from build123d import *

# Parameters (mm, degrees)
SKETCH1_W           = 72
SKETCH1_H           = 72
BOSS_EXTRUDE1_DEPTH = 15
SKETCH4_W           = 32
SKETCH4_H           = 64
CUT_EXTRUDE1_DEPTH  = 30
SKETCH8_R           = 10
SKETCH8_R_2         = 6
BOSS_EXTRUDE2_DEPTH = 10
BOSS_EXTRUDE3_DEPTH = 2


with BuildPart() as part:
    # Sketch1 → Boss-Extrude1 (new, symmetric)
    with BuildSketch(Plane.XY):
        with Locations((36, 36)):
            Rectangle(SKETCH1_W, SKETCH1_H)
    extrude(amount=BOSS_EXTRUDE1_DEPTH, both=True)

    # Sketch4 → Cut-Extrude1 (cut)
    with BuildSketch(Plane.XY.offset(15)):
        with Locations((56, 40)):
            Rectangle(SKETCH4_W, SKETCH4_H)
        with Locations((16, 40)):
            Rectangle(SKETCH4_W, SKETCH4_H)
    extrude(amount=-CUT_EXTRUDE1_DEPTH, mode=Mode.SUBTRACT)

    # Sketch8 → Boss-Extrude2 (add)
    with BuildSketch(Plane(origin=(0, 8, 0), x_dir=(1, 0, 0), z_dir=(0, 1, 0))):
        with Locations((18, 0)):
            Circle(SKETCH8_R)
        with Locations(Location((18, 0, 0), (0, 0, 180))):
            Circle(SKETCH8_R_2, mode=Mode.SUBTRACT)
    extrude(amount=BOSS_EXTRUDE2_DEPTH)

    # Sketch10 → Boss-Extrude3 (add, symmetric)
    with BuildSketch(Plane.XY):
        Polygon((40, 56), (54, 8), (72, 8), (72, 0), (0, 0), (0, 8), (32, 8), (32, 72), (40, 72), align=None)
    extrude(amount=BOSS_EXTRUDE3_DEPTH, both=True)


solid = part.part
CAD build for the part. Positions are in the model's coordinates, mm. A direction names the side the tool comes from. Give positions to 0.01 mm unless a question says otherwise; leave off trailing zeros. Loops run counter-clockwise (first coordinate to the right, second up) from the corner with the lowest first, then second, coordinate; pieces in that order, holes last. Notation, with made-up numbers: M -9.5,67.5 L 5.5,67.5 A18 cw 5.5,84.5 Z; hole C -1,-7.5 d8. An arc over 180 degrees is marked long. Write each question's results on one line, items separated by ' | '.
Q1. Band-saw the part on D-D on y = 61.5. Write the cut outline in (x, z).
Geometry check:
outline: M 32,-15 L 40,-15 L 40,15 L 32,15 Z
Q2. Band-saw the part on B-B on z = 0. Write the cut outline in (x, y).
Geometry check:
outline: M 0,0 L 72,0 L 72,8 L 54,8 L 40,56 L 40,72 L 32,72 L 32,8 L 28,8 L 28,18 L 24,18 L 24,8 L 12,8 L 12,18 L 8,18 L 8,8 L 0,8 Z
Q3. Band-saw the part on C-C on x = 18. Write the cut outline in (y, z).
Geometry check:
outline: M 0,-15 L 8,-15 L 8,-10 L 18,-10 L 18,-6 L 8,-6 L 8,6 L 18,6 L 18,10 L 8,10 L 8,15 L 0,15 Z
Q4. Flat gauge pins, fed straight in: P1, Ø9, axis at y = 53, z = -5, coming from the +X side; P2, Ø10, axis at y = 25.5, z = -2.5, coming from the -X side; P3, Ø8, axis at x = 63, z = 9.5, coming from the +Y side. Where does each tip first touch, or does it go through?
Geometry check:
P1: stops at x = 41.85 | P2: stops at x = 32 | P3: stops at y = 8
Q5. Which spindle directions (+Z, -Z, +X, -X, +Y, -Y) get a long thin tool onto all of the face, cutting with end or side? Do faces 4 (the face through (40, 40, 4)), 5 (the face through (25, 18, 0)), 6 (the face through (9, 8, 7)), 7 (the face through (44, 22, -2)). Say none if no direction does.
Geometry check:
face 4: +X, +Y | face 5: +Z, -Z, -X, +Y | face 6: +Y | face 7: -Z, +X, +Y
Q6. Band-saw the part on A-A on y = 17. Write the cut outline in (x, z) (3 decimals), and give its area (3 significant figures).
Geometry check:
outline: C 18,0 d20; M 32,-15 L 40,-15 L 40,-2 L 51.375,-2 L 51.375,2 L 40,2 L 40,15 L 32,15 Z; hole C 18,0 d12 | area: 487 mm²
Q7. Probe probe 1 along X at (y, z) = (10.25, 0); probe 2 along Y at (x, z) = (58, 7.5); probe 3 along X at (y, z) = (66.5, 1). List the from-to ranges inside material, lowest first.
Geometry check:
probe 1: x = 8 to 12, 24 to 28, 32 to 53.34 | probe 2: y = 0 to 8 | probe 3: x = 32 to 40
Q8. Mould opens along Z. For faces 1 (the face through (27.54, 12.93, -3)), 2 (the face through (24, 13, 0)), 3 (the face through (36, 20, -15)) say: pulls with the +Z half, pulls with the -Z half, needs draft (parallel to the pull), parting line crosses it, or undercut.
Geometry check:
face 1: parting line crosses it | face 2: undercut | face 3: pulls with the -Z half
